```python
from build123d import *

# Parameters (mm, degrees)
SKETCH1_W           = 3.175
SKETCH1_H           = 20
BOSS_EXTRUDE1_DEPTH = 400
SKETCH3_R           = 1.5
CUT_EXTRUDE1_DEPTH  = 400
SKETCH4_R           = 1.5
CUT_EXTRUDE2_DEPTH  = 400
FILLET1_R           = 0.5


with BuildPart() as part:
    # Sketch1 → Boss-Extrude1 (new body)
    with BuildSketch(Plane.XY):
        with Locations((1.5875, 10)):
            Rectangle(SKETCH1_W, SKETCH1_H)
        Polygon((0, 23.175), (0, 20), (3.175, 20), (23.175, 20), (23.175, 23.175), align=None)
    extrude(amount=BOSS_EXTRUDE1_DEPTH)

    # Sketch3 → Cut-Extrude1 (cut)
    with BuildSketch(Plane(origin=(0, 23.175, 0), x_dir=(1, 0, 0), z_dir=(0, 1, 0))):
        with Locations((13.175, -200)):
            Circle(SKETCH3_R)
        with Locations((13.175, -385)):
            Circle(SKETCH3_R)
        with Locations((13.175, -15)):
            Circle(SKETCH3_R)
    extrude(amount=-CUT_EXTRUDE1_DEPTH, mode=Mode.SUBTRACT)

    # Sketch4 → Cut-Extrude2 (cut)
    with BuildSketch(Plane(origin=(3.175, 0, 0), x_dir=(0, 0, -1), z_dir=(1, 0, 0))):
        with Locations((-385, 10)):
            Circle(SKETCH4_R)
        with Locations((-200, 10)):
            Circle(SKETCH4_R)
        with Locations((-15, 10)):
            Circle(SKETCH4_R)
    extrude(amount=-CUT_EXTRUDE2_DEPTH, mode=Mode.SUBTRACT)

    # Fillet1
    fillet1_edges = [part.edges().sort_by_distance(p)[0] for p in [
        (0, 23.175, 200),
        (3.175, 20, 200),
    ]]
    fillet(fillet1_edges, radius=FILLET1_R)


solid = part.part
```
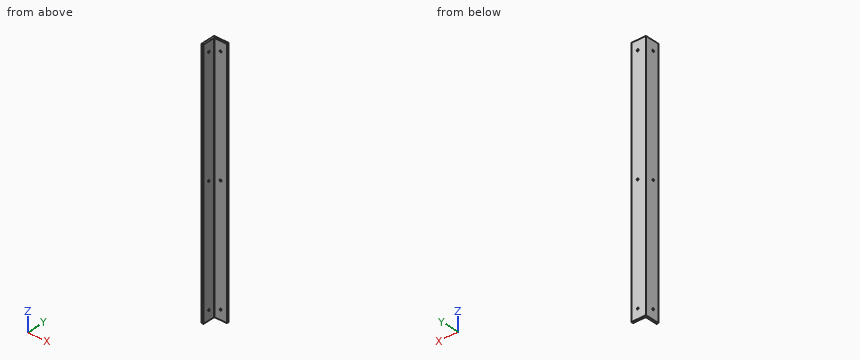
Here's how the part is built. I have some questions about the finished solid (model axes, mm). Give positions to 0.01 mm unless a question says otherwise; leave off trailing zeros. Order: outer loops, then holes, each group sorted by start corner. A loop starts at its lowest first (then second) coordinate and runs counter-clockwise, first axis right, second up. Notation, with made-up numbers: (88.5, 50) -> (138.5, 50) arc R22 cw to (138.5, 76) -> close; hole circle Ø7 at (-34.75, -30.75). An arc over 180 degrees is marked (long way). Use CSV: the item, a comma, the result in double quotes. Start each with the question number.
Item 1: Suppose I cut it at A-A (z = 164). List the corners of the cut face in (x, y) for me (3 decimals).
Item 2: Suppose I cut it at C-C (y = 14.75). List the corners of the cut face in (x, z) for me (3 decimals), and give its area (3 significant figures).
Item 3: If I drill on probe 1 along Z at (x, y) = (14, 21.5); probe 2 along Y at (x, z) = (1.75, 15) (3 decimals); probe 3 along X at (y, z) = (21.15, 200) (3 decimals), over which ranges is the centre line in solid material (lowest first)? Write a range as [from, to].
Item 4: Suppose I cut it at B-B (x = 7). List the corners of the cut face in (y, z) for me (3 decimals), and give its area (3 significant figures).
Item 5: I'm going to push flat-ended pins straight in: P1, Ø6, axis at x = 20.5, z = 254.5, coming from the -Y side; P2, Ø5, axis at y = 8.5, z = 172.5, coming from the +X side (3 decimals); P3, Ø3.5, axis at y = 10, z = 15, coming from the -X side. Where does each tip first touch, or does it pass through?
Answer block:
1,outline,"(0, 0) -> (3.175, 0) -> (3.175, 19.5) arc R0.5 cw to (3.675, 20) -> (23.175, 20) -> (23.175, 23.175) -> (0.5, 23.175) arc R0.5 ccw to (0, 22.675) -> close"
2,outline,"(0, 0) -> (3.175, 0) -> (3.175, 400) -> (0, 400) -> close"
2,area,"1,270 mm^2"
3,probe 1,"z = [0, 13.75], [16.25, 198.75], [201.25, 383.75], [386.25, 400]"
3,probe 2,"y = [0, 8.5], [11.5, 23.175]"
3,probe 3,"x = [0, 11.675], [14.675, 23.175]"
4,outline,"(20, 0) -> (23.175, 0) -> (23.175, 400) -> (20, 400) -> close"
4,area,"1,270 mm^2"
5,P1,"stops at y = 20"
5,P2,"stops at x = 3.175"
5,P3,"stops at x = 0"
